Input: part model. Units: mm. Frame: model coordinates. Face numbers are marked on the shaded views. Coordinates: 2 decimals unless noted, no trailing zeros. Order: outer loops, then holes, each group sorted by start corner. A loop starts at its lowest first (then second) coordinate and runs counter-clockwise, first axis right, second up. Notation, with made-up numbers: (10.25, -18) - (14.25, -18) arc R17 cw to (14.25, -3) - close; hole circle Ø10 at (13.25, -6.75). An arc over 180 degrees is marked (long way). One line per question, with ' | ' between items.
from build123d import *

# Parameters (mm, degrees)
SKETCH_1_R      = 1.25
SKETCH_1_R_2    = 2.5
SKETCH_1_R_3    = 1
EXTRUDE_1_DEPTH = 3
EXTRUDE_2_DEPTH = 1.75
FILLET_1_R      = 1.75


with BuildPart() as part:
    # 草图1 → 凸台-拉伸1 (new body)
    with BuildSketch(Plane.XY):
        with BuildLine():
            Line((0.75, 7.462405778), (25.5, 4.974937186))
            ThreePointArc((25.5, 4.974937186), (30, 0), (25.5, -4.974937186))
            Line((25.5, -4.974937186), (0.75, -7.462405778))
            ThreePointArc((0.75, -7.462405778), (-7.5, 0), (0.75, 7.462405778))
        make_face()
        with Locations((5, 0)):
            Circle(SKETCH_1_R, mode=Mode.SUBTRACT)
        with Locations((0, -5)):
            Circle(SKETCH_1_R, mode=Mode.SUBTRACT)
        with Locations((-5, 0)):
            Circle(SKETCH_1_R, mode=Mode.SUBTRACT)
        Circle(SKETCH_1_R_2, mode=Mode.SUBTRACT)
        with Locations((5.196152423, -3)):
            Circle(SKETCH_1_R_3, mode=Mode.SUBTRACT)
        with Locations((-5.196152423, -3)):
            Circle(SKETCH_1_R_3, mode=Mode.SUBTRACT)
        with BuildLine():
            ThreePointArc((-0.975780937, 5.78125), (0, 3.75), (0.975780937, 5.78125))
            ThreePointArc((0.975780937, 5.78125), (0, 7), (-0.975780937, 5.78125))
        make_face(mode=Mode.SUBTRACT)
    extrude(amount=EXTRUDE_1_DEPTH)

    # 草图2 → 凸台-拉伸2 (add, symmetric)
    with BuildSketch(Plane(origin=(25, 0, 0), x_dir=(0, 0, -1), z_dir=(1, 0, 0))):
        with BuildLine():
            Line((3, -1.75), (0, -1.75))
            Line((0, -1.75), (0, 1.75))
            Line((0, 1.75), (3, 1.75))
            ThreePointArc((3, 1.75), (4.149066665, 2.285818585), (4.47721163, 3.510472267))
            Line((4.47721163, 3.510472267), (7.924038765, 4.118240888))
            ThreePointArc((7.924038765, 4.118240888), (6.830222216, 0.036061952), (3, -1.75))
        make_face()
    extrude(amount=EXTRUDE_2_DEPTH, both=True)

    # 圆角1
    fillet_1_edges = [part.edges().sort_by_distance(p)[0] for p in [
        (23.25, 0, 0),
        (25, 1.75, 0),
        (23.25, -1.75, -1.5),
        (25, -1.75, 0),
        (23.25, 0.036061952, -6.830222216),
        (25, -1.75, -3),
        (23.25, 3.814356577, -6.200625197),
        (25, 4.118240888, -7.924038765),
        (23.25, 2.285818585, -4.149066665),
        (25, 3.510472267, -4.47721163),
        (23.25, 1.75, -1.5),
        (25, 1.75, -3),
        (26.75, 0, 0),
        (26.75, -1.75, -1.5),
        (26.75, 0.036061952, -6.830222216),
        (26.75, 3.814356577, -6.200625197),
        (26.75, 2.285818585, -4.149066665),
        (26.75, 1.75, -1.5),
    ]]
    fillet(fillet_1_edges, radius=FILLET_1_R - 0.0001)  # a hair under: the kernel refuses the full size


solid = part.part
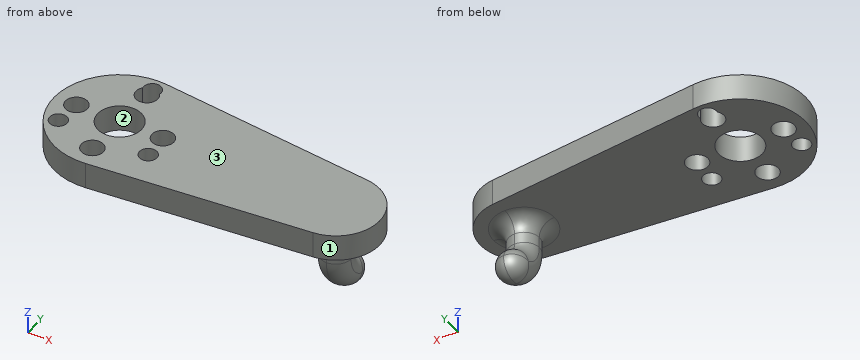
Item 1: Ray query, line 1 (Y direction, x = -5, z = 2); line 2 (Z direction, x = 5.5, y = 1.25); line 3 (Y direction, x = 25.5, z = 1.5). Return the intervals inside material, ascending.
Data:
line 1: -5.59 to -3.98, -2.02 to -1.25, 1.25 to 5.59 | line 2: 0 to 3 | line 3: -4.97 to 4.97
Item 2: Draft query along Y for the marked faces 1, 2 and 3. Return one class per face: released by +Y, released by -Y, zero draft, split by the parting line, or undercut.
Data:
face 1: split by the parting line | face 2: undercut | face 3: zero draft
Item 3: Section D-D on y = -3. Count the separate pieces of the cut face and the enclosed holes in it, and give its area (3 significant figures).
Data:
separate pieces: 3 | enclosed holes: 0 | area: 95.8 mm^2
Item 4: Section A-A on x = 0. Return the cut outline in (y, z), and give its area (4 significant figures).
Data:
outline: (-7.5, 0) - (-6.25, 0) - (-6.25, 3) - (-7.5, 3) - close; (-3.75, 0) - (-2.5, 0) - (-2.5, 3) - (-3.75, 3) - close; (2.5, 0) - (3.75, 0) - (3.75, 3) - (2.5, 3) - close; (7, 0) - (7.5, 0) - (7.5, 3) - (7, 3) - close | area: 12.75 mm^2
Item 5: Section C-C on z = 0.75. Return the cut outline in (x, y), and give its area (3 significant figures).
Data:
outline: (0.75, -7.46) - (25.5, -4.97) arc R5 ccw to (25.5, 4.97) - (0.75, 7.46) arc R7.5 ccw (long way) to start; hole circle Ø2.5 at (-5, 0); hole circle Ø2 at (-5.2, -3); hole circle Ø5 at (0, 0); hole circle Ø2.5 at (0, -5); hole (-0.98, 5.78) arc R1.25 ccw (long way) to (0.98, 5.78) arc R1 ccw (long way) to start; hole circle Ø2.5 at (5, 0); hole circle Ø2 at (5.2, -3) | area: 395 mm^2
Item 6: Section B-B on x = 5. Return the cut outline in (y, z).
Data:
outline: (-7.04, 0) - (-3.98, 0) - (-3.98, 3) - (-7.04, 3) - close; (-2.02, 0) - (-1.25, 0) - (-1.25, 3) - (-2.02, 3) - close; (1.25, 0) - (7.04, 0) - (7.04, 3) - (1.25, 3) - close
Item 7: Contact query for flat-ended pins moving along their axis: P1, Ø2, axis at x = 0, y = -5, coming from the -Z side; P2, Ø6, axis at y = 4, z = -6.5, coming from the -X side; P3, Ø0.6, axis at y = 0.5, z = -4, coming from the -X side; P4, Ø1, axis at x = 8, z = 2, coming from the +Y side. Output: stop coordinate, or through.
Data:
P1: through | P2: x = 23.25 | P3: x = 23.25 | P4: y = 6.78
